Part model, mm, in its own coordinate system. A direction names the side the tool comes from. Coordinates: 2 decimals unless noted, no trailing zeros. Write each loop counter-clockwise with the first axis right and the second up, starting at its lowest first coordinate (ties: lowest second). Pieces come first, ordered by that corner, then holes. Notation, with made-up numbers: (19, -28.5) -> (58, -28.5) arc R25 cw to (58, -4.5) -> close; hole circle Ø3 at (-19.75, -15.5). An arc over 180 degrees is marked (long way). One line per question, with ' | ' between items. Start each with the question number.
Item 1: Saw through at C-C (y = 12.25). List the corners of the cut face in (x, z).
Item 2: 3-axis set-ups, long thin cutter, end or side, ignore diameter. For faces 1 (the flat face through (13, 2, 15)), 2 (the flat face through (17, 7, 5)), 3 (the flat face through (10, 0, 8)), 4 (the flat face through (1, 16, 15)): which of +Z, -Z, +X, -X, +Y, -Y reach the whole face in a straight line?
Item 3: Saw through at B-B (x = 12.25). List the corners of the cut face in (y, z), and give its area (3 significant figures).
Item 4: Pin check, flat tips, straight feed: pin 1 (2 mm diameter, centred on y = 14.5, z = 17.5, fed in from +X); pin 2 (1.5 mm diameter, centred on y = 7, z = 17.5, fed in from +X); pin 3 (5 mm diameter, centred on x = 15, y = 16, fed in from +Z). Stop position of each tip, or through.
Item 5: Probe probe 1 along X at (y, z) = (7, 16.5); probe 2 along Y at (x, z) = (14.25, 13.75); probe 3 along X at (y, z) = (16, 2.75). List the from-to ranges inside material, lowest first. Write a range as [from, to].
Item 6: Saw through at D-D (x = 9.5). List the corners of the cut face in (y, z), and give its area (3 significant figures).
Item 7: Saw through at A-A (z = 2). List the corners of the cut face in (x, y), and give its area (3 significant figures).
from build123d import *

# Parameters (mm, degrees)
BOSS_EXTRUDE1_DEPTH = 20
SKETCH2_W           = 5
SKETCH2_H           = 20
BOSS_EXTRUDE2_DEPTH = 5
CUT_EXTRUDE1_DEPTH  = 21
BOSS_EXTRUDE4_DEPTH = 20
CUT_EXTRUDE2_DEPTH  = 70
SKETCH5_W           = 5
SKETCH5_H           = 10
BOSS_EXTRUDE5_DEPTH = 5
CUT_EXTRUDE3_DEPTH  = 5
BOSS_EXTRUDE6_DEPTH = 5
BOSS_EXTRUDE7_DEPTH = 5


with BuildPart() as part:
    # Sketch1 → Boss-Extrude1 (new body)
    with BuildSketch(Plane(origin=(0, 0, 0), x_dir=(1, 0, 0), z_dir=(0, 1, 0))):
        Polygon((0, -15), (0, 0), (10, 0), (10, -5), align=None)
    extrude(amount=BOSS_EXTRUDE1_DEPTH)

    # Sketch2 → Boss-Extrude2 (add)
    with BuildSketch(Plane(origin=(10, 0, 0), x_dir=(0, 0, -1), z_dir=(1, 0, 0))):
        with Locations((-2.5, 10)):
            Rectangle(SKETCH2_W, SKETCH2_H)
    extrude(amount=BOSS_EXTRUDE2_DEPTH)

    # Sketch3 → Cut-Extrude1 (cut)
    with BuildSketch(Plane(origin=(0, 0, 0), x_dir=(-1, 0, 0), z_dir=(0, 0, -1))):
        Polygon((-10, 20), (-15, 20), (-15, 15), align=None)
    extrude(amount=-CUT_EXTRUDE1_DEPTH, mode=Mode.SUBTRACT)

    # Sketch4 → Boss-Extrude4 (add)
    with BuildSketch(Plane(origin=(0, 0, 0), x_dir=(-1, 0, 0), z_dir=(0, -1, 0))):
        Polygon((0, -15), (-10, -5), (-15, -5), (-15, -10), (-10, -15), align=None)
    extrude(amount=-BOSS_EXTRUDE4_DEPTH)

    # 3DSketch1 → Cut-Extrude2 (cut, along a direction that is not the sketch's normal)
    with BuildSketch(Plane(origin=(0, 20, 15), x_dir=(0.8017837257372734, -0.26726124191242434, -0.5345224838248487), z_dir=(-0.5773502691896257, -0.5773502691896256, -0.5773502691896261))):
        Polygon((0, 0), (13.363062096, -4.629100499), (18.708286934, 0), (17.371980724, 6.943650748), (10.690449676, 9.258200998), align=None)
    extrude(amount=-CUT_EXTRUDE2_DEPTH, dir=(-1, 0, 0), mode=Mode.SUBTRACT)

    # Sketch5 → Boss-Extrude5 (add)
    with BuildSketch(Plane(origin=(15, 0, 0), x_dir=(0, 0, -1), z_dir=(1, 0, 0))):
        with Locations((-2.5, 5)):
            Rectangle(SKETCH5_W, SKETCH5_H)
    extrude(amount=BOSS_EXTRUDE5_DEPTH)

    # Sketch6 → Cut-Extrude3 (cut)
    with BuildSketch(Plane.XY.offset(5)):
        Polygon((15, 10), (20, 5), (20, 10), align=None)
    extrude(amount=-CUT_EXTRUDE3_DEPTH, mode=Mode.SUBTRACT)

    # Sketch7 → Boss-Extrude6 (add)
    with BuildSketch(Plane(origin=(0, 0, 0), x_dir=(-1, 0, 0), z_dir=(0, -1, 0))):
        Polygon((-15, -10), (-15, -5), (-20, -5), (-20, -10), (-15, -15), (-10, -15), align=None)
    extrude(amount=-BOSS_EXTRUDE6_DEPTH)

    # Sketch8 → Boss-Extrude7 (add)
    with BuildSketch(Plane.XY.offset(15)):
        Polygon((0, 15), (5, 15), (10, 10), (10, 0), (0, 0), align=None)
    extrude(amount=BOSS_EXTRUDE7_DEPTH)


solid = part.part
From the geometry:
1) outline: (0, 0) -> (15, 0) -> (15, 7.75) -> (7.75, 15) -> (7.75, 20) -> (0, 20) -> close
2) face 1: +Z, +X, +Y, -Y | face 2: +Z, +X, +Y | face 3: +Z, -Z, +X, -X, -Y | face 4: +Z, +X, -X, +Y
3) outline: (0, 0) -> (17.75, 0) -> (17.75, 5) -> (10, 12.75) -> (5, 12.75) -> (5, 15) -> (0, 15) -> close | area: 208 mm2
4) pin 1: x = 6.5 | pin 2: x = 10 | pin 3: z = 7.54
5) probe 1: [0, 10] | probe 2: [0, 5] | probe 3: [0, 14]
6) outline: (0, 0) -> (20, 0) -> (20, 5.5) -> (10.5, 15) -> (10.5, 20) -> (0, 20) -> close | area: 307 mm2
7) outline: (0, 0) -> (20, 0) -> (20, 5) -> (15, 10) -> (15, 15) -> (10, 20) -> (0, 20) -> close | area: 325 mm2
